Check sheet for the drawn part. Datum: minimum x, y, z corner. Units: mm. Round coordinates to 2 decimals unless told otherwise and drop trailing zeros. Write each loop counter-clockwise with the first axis right and the second up, starting at its lowest first coordinate (ties: lowest second). Pieces come first, ordered by that corner, then holes.
Item 1: Cross-section at C-C on z = 0.9. Count the separate pieces of the cut face and the enclosed holes in it, plus the area to 3 significant figures.
Item 2: Cross-section at B-B on x = 3. Enter the section's corners in (y, z).
Item 3: Cross-section at A-A on y = 2.9. Enter the section's corners in (x, z).
Item 4: Material ranges on line 1 (Y direction, x = 2.5, z = 0.55); line 2 (X direction, y = 3.2, z = 0.8); line 3 (X direction, y = 2.35, z = 1.7) (1 decimal), recorded low to high.
Item 5: Release check for a two-part mould opening along X. For the marked faces 1, 2, 3 and 4 record: +X half, -X half, draft (parallel to the pull), parting line (faces both ways), or undercut.
Item 6: Go/stop test with a flat-tipped pin: pin 1 Ø1 at (y, z) = (4, 2) entering from +X. Record where the tip stops, or that it passes through.
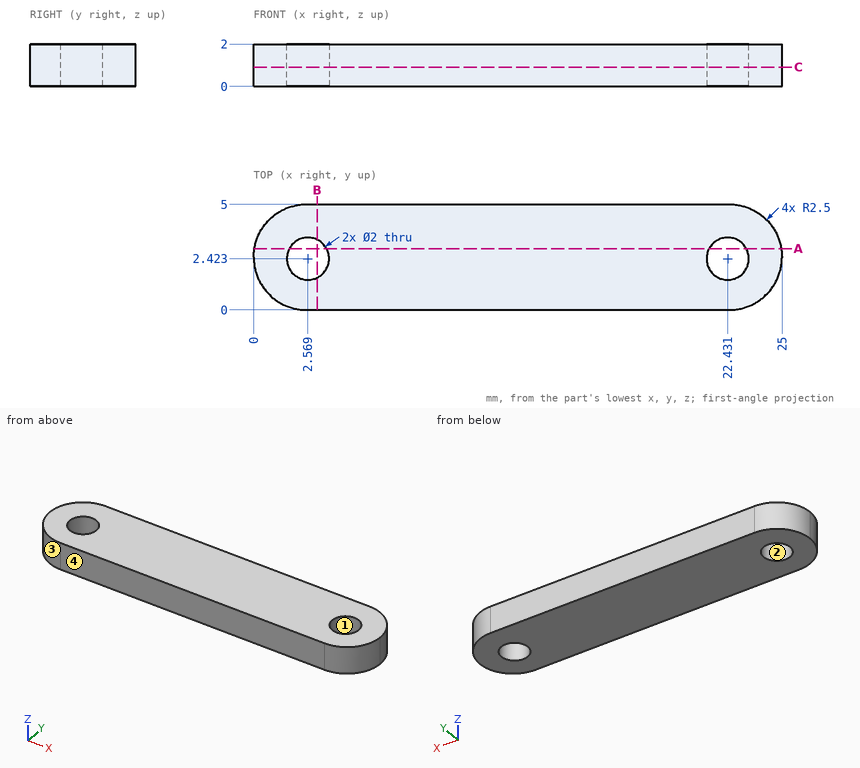
Response values:
1. separate pieces: 1
1. enclosed holes: 2
1. area: 113 mm2
2. outline: (0, 0) - (1.52, 0) - (1.52, 2) - (0, 2) - close; (3.33, 0) - (5, 0) - (5, 2) - (3.33, 2) - close
3. outline: (0.03, 0) - (1.69, 0) - (1.69, 2) - (0.03, 2) - close; (3.45, 0) - (21.55, 0) - (21.55, 2) - (3.45, 2) - close; (23.31, 0) - (24.97, 0) - (24.97, 2) - (23.31, 2) - close
4. line 1: y = 0 to 1.43, 3.42 to 5
4. line 2: x = 0.1 to 1.94, 3.2 to 21.8, 23.06 to 24.9
4. line 3: x = 0 to 1.6, 3.6 to 21.4, 23.4 to 25
5. face 1: undercut
5. face 2: undercut
5. face 3: -X half
5. face 4: draft
6. pin 1: stops at x = 24.79
